The model under review builds one solid part; all positions refer to its coordinate system, in mm. Face numbers are marked on the shaded views. A direction names the side the tool comes from. Coordinates: 2 decimals unless noted, no trailing zeros. Write each loop counter-clockwise with the first axis right and the second up, starting at its lowest first coordinate (ties: lowest second). Pieces come first, ordered by that corner, then holes. Notation, with made-up numbers: (52, -10) - (97, -10) arc R15 ccw to (97, 12) - close; hole circle Ø7 at (12, 52). An arc over 180 degrees is marked (long way). Return JSON: item names as keys, results as strings. Group by question number.
(1) To check wall thickness, follow L1, parallel to X at y = -3, z = 6.5; L2, parallel to X at y = 26, z = 25; L3, parallel to Z at x = 46, y = 26. State the ranges of each line that lie inside material, in increasing order. Write a range as from..to.
(2) We need section D-D on x = 8.5. State the section outline as (y, z) points.
(3) For pin 1 Ø3 at (x, y) = (-5, 24.5) entering from +Z; pin 2 Ø1.2 at (x, z) = (50.05, 21) entering from -Y; pin 3 Ø4 at (y, z) = (-5.5, 13.5) entering from +X; pin 4 Ø6 at (x, z) = (40, 13) entering from -Y, all flat-tipped, find the tip position at first contact; note any pin that passes through.
(4) We need section B-B on z = 18. Give the number of separate pieces and of enclosed holes in the cut face, then the cut area to 3 significant figures.
(5) Tool access review of the marked faces 1, 2, 3 and 4: name each direction out of +Z, -Z, +X, -X, +Y, -Y from which nothing blocks a thin tool from reaching the whole face with its end or side.
(6) Draft analysis for pull direction X (two halves, no side actions). For the marked faces 5, 6 and 7, state which applies: released by +X, released by -X, zero draft, split by the parting line, or undercut.
(7) We need section A-A on y = -4. State the section outline as (x, z) points.
(8) We need section C-C on x = 36.05. State the section outline as (y, z) points, then the cut area to 3 significant figures.
```python
from build123d import *

# Parameters (mm, degrees)
SKETCH1_W           = 26.1
SKETCH1_H           = 46.1
SKETCH1_W_2         = 20.1
SKETCH1_H_2         = 40.1
BOSS_EXTRUDE1_DEPTH = 31
SKETCH2_W           = 26.1
SKETCH2_H           = 46.1
BOSS_EXTRUDE2_DEPTH = 3
SKETCH3_R           = 10
BOSS_EXTRUDE3_DEPTH = 2
SKETCH4_W           = 26.1
SKETCH4_H           = 3.95
SKETCH4_R           = 0.836516838
BOSS_EXTRUDE4_DEPTH = 5
SKETCH5_W           = 26
SKETCH5_H           = 3
BOSS_EXTRUDE5_DEPTH = 5
SKETCH7_W           = 26
SKETCH7_H           = 55.2
BOSS_EXTRUDE6_DEPTH = 5
BOSS_EXTRUDE7_DEPTH = 55.2
SKETCH9_R           = 2.5
SKETCH9_R_2         = 1
CUT_EXTRUDE1_DEPTH  = 13.2
SKETCH10_R          = 10.025
CUT_EXTRUDE2_DEPTH  = 13.2
SKETCH11_W          = 37.335387761
SKETCH11_H          = 47.2
CUT_EXTRUDE3_DEPTH  = 43.2
SKETCH12_R          = 10.025
CUT_EXTRUDE4_DEPTH  = 2.8
SKETCH13_W          = 6
SKETCH13_H          = 4
CUT_EXTRUDE5_DEPTH  = 24


with BuildPart() as part:
    # Sketch1 → Boss-Extrude1 (new body)
    with BuildSketch(Plane.XY):
        Rectangle(SKETCH1_W, SKETCH1_H)
        Rectangle(SKETCH1_W_2, SKETCH1_H_2, mode=Mode.SUBTRACT)
    extrude(amount=BOSS_EXTRUDE1_DEPTH)

    # Sketch2 → Boss-Extrude2 (add)
    with BuildSketch(Plane.XY.offset(31)):
        Rectangle(SKETCH2_W, SKETCH2_H)
    extrude(amount=-BOSS_EXTRUDE2_DEPTH)

    # Sketch3 → Boss-Extrude3 (add)
    with BuildSketch(Plane.XY.offset(31)):
        with Locations((-0.05, 10.05)):
            Circle(SKETCH3_R)
    extrude(amount=BOSS_EXTRUDE3_DEPTH)

    # Sketch4 → Boss-Extrude4 (add)
    with BuildSketch(Plane(origin=(0, 0, 0), x_dir=(-1, 0, 0), z_dir=(0, 0, -1))):
        with Locations((0, 25.025)):
            Rectangle(SKETCH4_W, SKETCH4_H)
        with Locations((-5, 24.4)):
            Circle(SKETCH4_R, mode=Mode.SUBTRACT)
        with Locations((5, 24.4)):
            Circle(SKETCH4_R, mode=Mode.SUBTRACT)
    boss_extrude4 = extrude(amount=-BOSS_EXTRUDE4_DEPTH)

    # Mirror1: Boss-Extrude4 across plane
    add(boss_extrude4.mirror(Plane.ZX))

    # Sketch5 → Boss-Extrude5 (add)
    with BuildSketch(Plane(origin=(13.05, 0, 0), x_dir=(0, 0, -1), z_dir=(1, 0, 0))):
        with Locations((-18, 20)):
            Rectangle(SKETCH5_W, SKETCH5_H)
        with Locations((-18, 10)):
            Rectangle(SKETCH5_W, SKETCH5_H)
        with Locations((-18, 0)):
            Rectangle(SKETCH5_W, SKETCH5_H)
        with Locations((-18, -10)):
            Rectangle(SKETCH5_W, SKETCH5_H)
        with Locations((-18, -20)):
            Rectangle(SKETCH5_W, SKETCH5_H)
    extrude(amount=BOSS_EXTRUDE5_DEPTH)

    # Sketch7 → Boss-Extrude6 (add)
    with BuildSketch(Plane(origin=(18.05, 0, 0), x_dir=(0, 0, -1), z_dir=(1, 0, 0))):
        with Locations((-18, -0.05)):
            Rectangle(SKETCH7_W, SKETCH7_H)
    extrude(amount=BOSS_EXTRUDE6_DEPTH)

    # Sketch8 → Boss-Extrude7 (add)
    with BuildSketch(Plane(origin=(0, 27.55, 0), x_dir=(1, 0, 0), z_dir=(0, 1, 0))):
        with BuildLine():
            Line((43.640549012, -6.014539981), (23.05, -5))
            Line((23.05, -5), (23.05, -31))
            Line((23.05, -31), (43.640549012, -29.985460019))
            ThreePointArc((43.640549012, -29.985460019), (55.05, -18), (43.640549012, -6.014539981))
        make_face()
    extrude(amount=-BOSS_EXTRUDE7_DEPTH)

    # Sketch9 → Cut-Extrude1 (cut)
    with BuildSketch(Plane(origin=(0, 27.55, 0), x_dir=(1, 0, 0), z_dir=(0, 1, 0))):
        with Locations(Location((43.05, -18, 0), (0, 0, 270))):
            Circle(SKETCH9_R)
        with Locations(Location((50.05, -15, 0), (0, 0, 270))):
            Circle(SKETCH9_R_2)
        with Locations(Location((50.05, -18, 0), (0, 0, 270))):
            Circle(SKETCH9_R_2)
        with Locations(Location((50.05, -21, 0), (0, 0, 270))):
            Circle(SKETCH9_R_2)
        with Locations(Location((46.05, -25, 0), (0, 0, 270))):
            Circle(SKETCH9_R_2)
        with Locations(Location((43.05, -25, 0), (0, 0, 270))):
            Circle(SKETCH9_R_2)
        with Locations(Location((40.05, -25, 0), (0, 0, 270))):
            Circle(SKETCH9_R_2)
        with Locations(Location((36.05, -21, 0), (0, 0, 270))):
            Circle(SKETCH9_R_2)
        with Locations(Location((36.05, -18, 0), (0, 0, 270))):
            Circle(SKETCH9_R_2)
        with Locations(Location((36.05, -15, 0), (0, 0, 270))):
            Circle(SKETCH9_R_2)
        with Locations(Location((40.05, -11, 0), (0, 0, 270))):
            Circle(SKETCH9_R_2)
        with Locations(Location((43.05, -11, 0), (0, 0, 270))):
            Circle(SKETCH9_R_2)
        with Locations(Location((46.05, -11, 0), (0, 0, 270))):
            Circle(SKETCH9_R_2)
    extrude(amount=-CUT_EXTRUDE1_DEPTH, mode=Mode.SUBTRACT)

    # Sketch10 → Cut-Extrude2 (cut)
    with BuildSketch(Plane.XZ.offset(27.65)):
        with Locations(Location((43.05, 18, 0), (0, 0, 270))):
            Circle(SKETCH10_R)
    extrude(amount=-CUT_EXTRUDE2_DEPTH, mode=Mode.SUBTRACT)

    # Sketch11 → Cut-Extrude3 (cut)
    with BuildSketch(Plane(origin=(0, 0, 5), x_dir=(-1, 0, 0), z_dir=(0, 0, -1))):
        with Locations((-41.717693881, -1.05)):
            Rectangle(SKETCH11_W, SKETCH11_H)
    extrude(amount=-CUT_EXTRUDE3_DEPTH, mode=Mode.SUBTRACT)

    # Sketch12 → Cut-Extrude4 (cut)
    with BuildSketch(Plane.XZ.offset(-22.55)):
        with Locations(Location((43.05, 18, 0), (0, 0, 270))):
            Circle(SKETCH12_R)
    extrude(amount=-CUT_EXTRUDE4_DEPTH, mode=Mode.SUBTRACT)

    # Sketch13 → Cut-Extrude5 (cut)
    with BuildSketch(Plane(origin=(0, 0, 0), x_dir=(-1, 0, 0), z_dir=(0, 0, -1))):
        with Locations((0, 22.05)):
            Rectangle(SKETCH13_W, SKETCH13_H)
    extrude(amount=-CUT_EXTRUDE5_DEPTH, mode=Mode.SUBTRACT)


solid = part.part
```
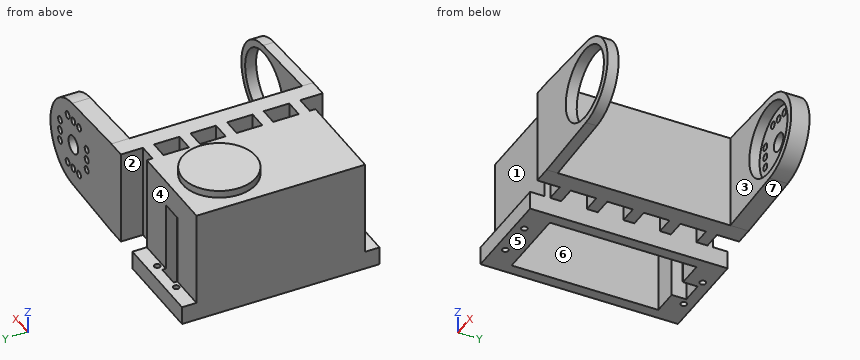
Ans:
{
 "1": {"L1": "-13.05..-10.05, 10.05..13.05, 18.05..23.05", "L2": "18.05..39.05, 41.05..42.05, 44.05..45.05, 47.05..52.8", "L3": "6.37..10, 12..24, 26..29.63"},
 "2": {"outline": "(-27, 0) - (-20.05, 0) - (-20.05, 28) - (20.05, 28) - (20.05, 0) - (27, 0) - (27, 5) - (23.05, 5) - (23.05, 31) - (15.24, 31) - (15.24, 33) - (4.86, 33) - (4.86, 31) - (-23.05, 31) - (-23.05, 5) - (-27, 5) - close"},
 "3": {"pin 1": "z = 31", "pin 2": "through", "pin 3": "x = 23.05", "pin 4": "y = 25.35"},
 "4": {"separate pieces": "5", "enclosed holes": "4", "area": "850 mm²"},
 "5": {"face 1": "+Z, -X, -Y", "face 2": "+Z, -Z, +Y", "face 3": "+Z, -Z, +X", "face 4": "+Z, -X, +Y"},
 "6": {"face 5": "zero draft", "face 6": "undercut", "face 7": "released by +X"},
 "7": {"outline": "(-13.05, 0) - (-10.05, 0) - (-10.05, 28) - (10.05, 28) - (10.05, 0) - (13.05, 0) - (13.05, 31) - (-13.05, 31) - close; (18.05, 5) - (23.05, 5) - (23.05, 31) - (18.05, 31) - close"},
 "8": {"outline": "(-27.65, 5.64) - (-24.65, 5.64) - (-24.65, 10.82) - (-27.65, 10.82) - close; (-27.65, 25.18) - (-24.65, 25.18) - (-24.65, 30.36) - (-27.65, 30.36) - close; (22.55, 5.64) - (27.55, 5.64) - (27.55, 14) - (25.35, 14) - (25.35, 10.82) - (22.55, 10.82) - close; (22.55, 25.18) - (25.35, 25.18) - (25.35, 22) - (27.55, 22) - (27.55, 30.36) - (22.55, 30.36) - close; (25.35, 16) - (27.55, 16) - (27.55, 17) - (25.35, 17) - close; (25.35, 19) - (27.55, 19) - (27.55, 20) - (25.35, 20) - close", "area": "101 mm²"}
}
